The listing builds one solid part. Answer for the finished solid, in the listing's coordinates (mm). A direction names the side the tool comes from. Round coordinates to 2 decimals unless told otherwise and drop trailing zeros. Loops run counter-clockwise (first coordinate to the right, second up) from the corner with the lowest first, then second, coordinate; pieces in that order, holes last. Notation, with made-up numbers: M 27.5,20 L 31.5,20 A17 ccw 31.5,49 Z; hole C -38,34 d5. An arc over 180 degrees is marked long. Answer as a JSON object with one key per item and string values.
```python
from build123d import *

# Parameters (mm, degrees)
SKETCH1_W             = 32.708231768
SKETCH1_H             = 10.82386404
SKETCH1_W_2           = 30
SKETCH1_H_2           = 3.5
BOSS_EXTRUDE2_DEPTH   = 15
SKETCH4_W             = 47
SKETCH4_H             = 15.552838856
SKETCH4_W_2           = 30
SKETCH4_H_2           = 3.5
BOSS_EXTRUDE4_DEPTH   = 4
SKETCH7_W             = 47
SKETCH7_H             = 15.5
SKETCH7_W_2           = 30
SKETCH7_H_2           = 3.5
BOSS_EXTRUDE5_DEPTH   = 5.782
SKETCH25_W            = 47
SKETCH25_H            = 5.782
BOSS_EXTRUDE9_DEPTH   = 5.175
M3X0_5_TAPPED_HOLE1_D = 2.5
FILLET5_R             = 2
SKETCH26_W            = 47
SKETCH26_H            = 4
BOSS_EXTRUDE10_DEPTH  = 5.175
SKETCH17_W            = 47
SKETCH17_H            = 3.015322823
BOSS_EXTRUDE7_DEPTH   = 20.76
M3X0_5_TAPPED_HOLE2_D = 2.5
FILLET6_R             = 1
FILLET8_R             = 1
FILLET9_R             = 1
FILLET10_R            = 1


with BuildPart() as part:
    # Sketch1 → Boss-Extrude2 (new body)
    with BuildSketch(Plane(origin=(0, 0, 0), x_dir=(1, 0, 0), z_dir=(0, 1, 0))):
        Rectangle(SKETCH1_W, SKETCH1_H)
        Rectangle(SKETCH1_W_2, SKETCH1_H_2, mode=Mode.SUBTRACT)
    extrude(amount=BOSS_EXTRUDE2_DEPTH)

    # Sketch4 → Boss-Extrude4 (add)
    with BuildSketch(Plane(origin=(0, 15, 0), x_dir=(1, 0, 0), z_dir=(0, 1, 0))):
        Rectangle(SKETCH4_W, SKETCH4_H)
        Rectangle(SKETCH4_W_2, SKETCH4_H_2, mode=Mode.SUBTRACT)
    extrude(amount=BOSS_EXTRUDE4_DEPTH)

    # Sketch7 → Boss-Extrude5 (add)
    with BuildSketch(Plane.XZ):
        Rectangle(SKETCH7_W, SKETCH7_H)
        Rectangle(SKETCH7_W_2, SKETCH7_H_2, mode=Mode.SUBTRACT)
    extrude(amount=BOSS_EXTRUDE5_DEPTH)

    # Sketch25 → Boss-Extrude9 (add)
    with BuildSketch(Plane(origin=(0, 0, -7.75), x_dir=(-1, 0, 0), z_dir=(0, 0, -1))):
        with Locations((0, -2.891)):
            Rectangle(SKETCH25_W, SKETCH25_H)
    extrude(amount=BOSS_EXTRUDE9_DEPTH)

    # M3x0.5 Tapped Hole1 (through all)
    with Locations(Plane(origin=(0, 0, 7.75), x_dir=(-1, 0, 0), z_dir=(0, 0, 1))):
        with Locations((20.12, 2.891216796), (-20.12, 2.891216796)):
            Hole(M3X0_5_TAPPED_HOLE1_D / 2)

    # Fillet5
    fillet5_edges = [part.edges().sort_by_distance(p)[0] for p in [
        (16.354115884, 7.5, 5.41193202),
        (-16.354115884, 7.5, 5.41193202),
        (-16.354115884, 7.5, -5.41193202),
        (16.354115884, 7.5, -5.41193202),
    ]]
    fillet(fillet5_edges, radius=FILLET5_R)

    # Sketch26 → Boss-Extrude10 (add)
    with BuildSketch(Plane(origin=(0, 0, -7.776419428), x_dir=(-1, 0, 0), z_dir=(0, 0, -1))):
        with Locations((0, 17)):
            Rectangle(SKETCH26_W, SKETCH26_H)
    extrude(amount=BOSS_EXTRUDE10_DEPTH)

    # Sketch17 → Boss-Extrude7 (add)
    with BuildSketch(Plane(origin=(0, 19, 0), x_dir=(1, 0, 0), z_dir=(0, 1, 0))):
        with Locations((0, 11.443758017)):
            Rectangle(SKETCH17_W, SKETCH17_H)
    extrude(amount=BOSS_EXTRUDE7_DEPTH)

    # M3x0.5 Tapped Hole2 (through all)
    with Locations(Plane(origin=(0, 0, -12.951419428), x_dir=(-1, 0, 0), z_dir=(0, 0, -1))):
        with Locations((-4.7, 35.51), (4.7, 35.51)):
            Hole(M3X0_5_TAPPED_HOLE2_D / 2)

    # Fillet6
    fillet6_edges = [part.edges().sort_by_distance(p)[0] for p in [
        (-23.5, 39.76, -11.443758016),
    ]]
    fillet(fillet6_edges, radius=FILLET6_R)

    # Fillet8
    fillet8_edges = [part.edges().sort_by_distance(p)[0] for p in [
        (23.5, 39.76, -11.443758016),
        (23.5, -5.782, -2.5875),
        (-23.5, -5.782, -2.5875),
        (23.5, 0, -2.5875),
        (-23.5, 0, -2.5875),
    ]]
    fillet(fillet8_edges, radius=FILLET8_R)

    # Fillet9
    fillet9_edges = [part.edges().sort_by_distance(p)[0] for p in [
        (-23.5, 15, -2.5875),
    ]]
    fillet(fillet9_edges, radius=FILLET9_R)

    # Fillet10
    fillet10_edges = [part.edges().sort_by_distance(p)[0] for p in [
        (23.5, 15, -2.5875),
    ]]
    fillet(fillet10_edges, radius=FILLET10_R)


solid = part.part
```
Item 1: Determine the mould class of faces 4 (the face through (0, 17, 7.776)), 5 (the face through (-15.753, 7.605, 4.842)), 6 (the face through (19.2, -3.74, -2.73)), 7 (the face through (15.753, 7.605, 4.842)) for opening direction X: released by +X, released by -X, zero draft, split by the parting line, or undercut.
Values follow:
{"face 4": "zero draft", "face 5": "released by -X", "face 6": "undercut", "face 7": "released by +X"}
Item 2: Straight lines are drawn through the part: line 1 (Y direction, x = -20.12, z = -1.5); line 2 (Y direction, x = 4.7, z = -10.6); line 3 (X direction, y = 14.5, z = 0.25). For each, find the intervals that lie inside material, in ascending order.
Values follow:
{"line 1": "-5.78 to -4.14, -1.64 to 0, 15 to 19", "line 2": "-5.78 to 0, 15 to 34.26, 36.76 to 39.76", "line 3": "-16.35 to -15, 15 to 16.35"}
Item 3: Flat-ended cylindrical pins translate along their axes: P1, Ø1, axis at x = -18.5, y = 6, coming from the +Z side; P2, Ø5.5, axis at y = 9.5, z = 0, coming from the +X side; P3, Ø1.5, axis at x = -3.5, y = 7, coming from the +Z side; P4, Ø6, axis at x = -9, z = 0, coming from the -Y side. Find the tip coordinate at first contact, or state that the pin passes through.
Values follow:
{"P1": "through", "P2": "x = 16.35", "P3": "z = 5.41", "P4": "y = -5.78"}
Item 4: The part is cut by section B-B (y = 35.51). Give the vertices of the cut face in (x, z).
Values follow:
{"outline": "M -23.5,-12.95 L -5.95,-12.95 L -5.95,-9.94 L -23.5,-9.94 Z; M -3.45,-12.95 L 3.45,-12.95 L 3.45,-9.94 L -3.45,-9.94 Z; M 5.95,-12.95 L 23.5,-12.95 L 23.5,-9.94 L 5.95,-9.94 Z"}
Item 5: The part is cut by section C-C (z = -7). Give the vertices of the cut face in (x, y), then the cut area to 3 significant figures.
Values follow:
{"outline": "M -23.5,-4.78 A1 ccw -22.5,-5.78 L 22.5,-5.78 A1 ccw 23.5,-4.78 L 23.5,-1 A1 ccw 22.5,0 L -22.5,0 A1 ccw -23.5,-1 Z; M -23.5,16 A1 ccw -22.5,15 L 22.5,15 A1 ccw 23.5,16 L 23.5,19 L -23.5,19 Z; hole C -20.12,-2.89 d2.5; hole C 20.12,-2.89 d2.5", "area": "449 mm^2"}
Item 6: The part is cut by section D-D (z = -10.5). Give the vertices of the cut face in (x, y).
Values follow:
{"outline": "M -23.5,-4.78 A1 ccw -22.5,-5.78 L 22.5,-5.78 A1 ccw 23.5,-4.78 L 23.5,-1 A1 ccw 22.5,0 L -22.5,0 A1 ccw -23.5,-1 Z; M -23.5,16 A1 ccw -22.5,15 L 22.5,15 A1 ccw 23.5,16 L 23.5,38.76 A1 ccw 22.5,39.76 L -22.5,39.76 A1 ccw -23.5,38.76 Z; hole C -20.12,-2.89 d2.5; hole C -4.7,35.51 d2.5; hole C 4.7,35.51 d2.5; hole C 20.12,-2.89 d2.5"}
Item 7: Which of the six approach directions +Z, -Z, +X, -X, +Y, -Y give full straight-line access (tool end or side, diameter ignored) to faces 1 (the face through (0, 7, -5.412)), 2 (the face through (0, 29, -9.936)), 3 (the face through (15, 7, 0))?
Values follow:
{"face 1": "-Z, +X, -X", "face 2": "+Z, +X, -X, +Y", "face 3": "+Y, -Y"}
Item 8: The part is cut by section A-A (x = 4.7). Give the vertices of the cut face in (y, z) (3 decimals).
Values follow:
{"outline": "M -5.782,-12.925 L 0,-12.925 L 0,-5.412 L 15,-5.412 L 15,-12.951 L 34.26,-12.951 L 34.26,-9.936 L 19,-9.936 L 19,-1.75 L -5.782,-1.75 Z; M -5.782,1.75 L 19,1.75 L 19,7.776 L 15,7.776 L 15,5.412 L 0,5.412 L 0,7.75 L -5.782,7.75 Z; M 36.76,-12.951 L 39.76,-12.951 L 39.76,-9.936 L 36.76,-9.936 Z"}
